Source: three-view drawing plus pictorial views. Frame: mm from the lowest corner of the part. A direction names the side the tool comes from. Give positions to 0.01 mm unless a question says otherwise; leave off trailing zeros. Loops run counter-clockwise (first coordinate to the right, second up) from the corner with the lowest first, then second, coordinate; pieces in that order, holes last. Notation, with made-up numbers: (22.5, -27) - (57.5, -27) arc R15 ccw to (57.5, -14) - close; hole circle Ø2 at (44.5, 10.25). An arc over 180 degrees is marked (long way). One line per item, written item: value.
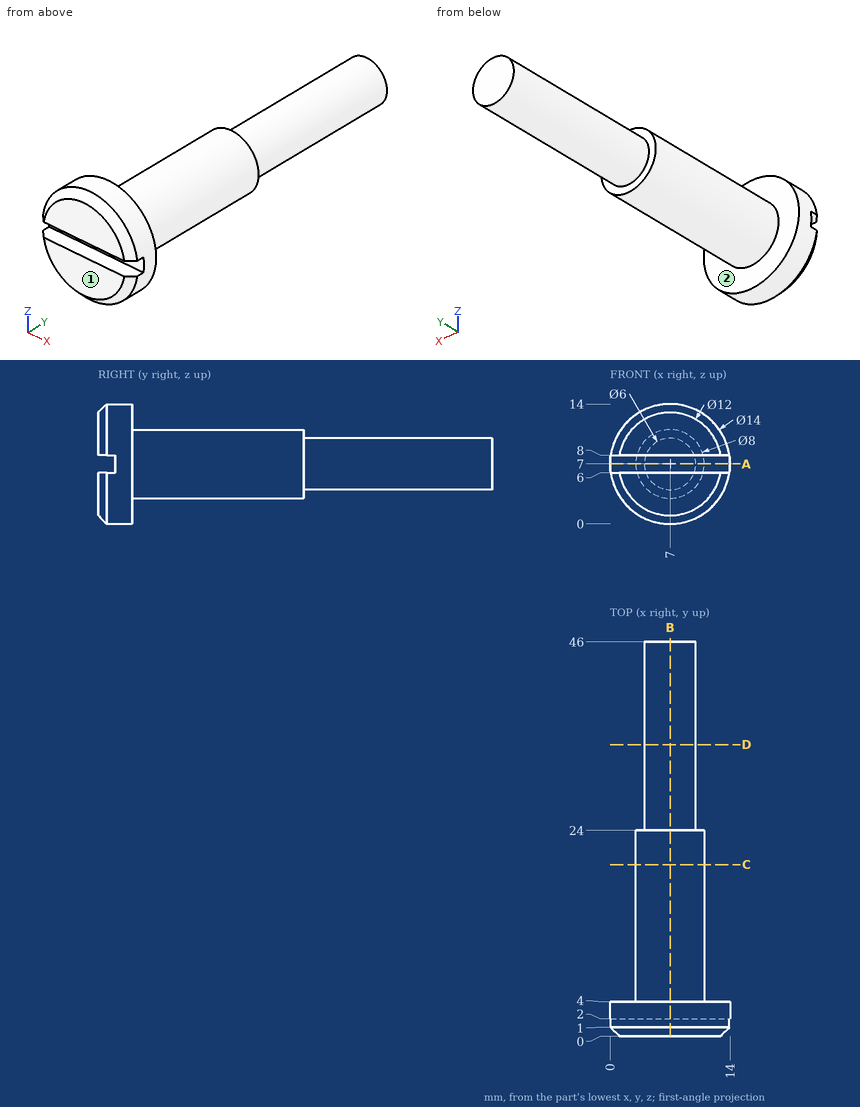
Item 1: Section C-C, the plane y = 20. Output: boundary loops of the cut face in (x, z).
Verdict:
outline: circle Ø8 at (7, 7)
Item 2: Section B-B, the plane x = 7. Output: boundary loops of the cut face in (y, z), and give its area (3 significant figures).
Verdict:
outline: (0, 1) - (1, 0) - (4, 0) - (4, 3) - (24, 3) - (24, 4) - (46, 4) - (46, 10) - (24, 10) - (24, 11) - (4, 11) - (4, 14) - (1, 14) - (0, 13) - (0, 8) - (2, 8) - (2, 6) - (0, 6) - close
area: 343 mm^2
Item 3: Section A-A, the plane z = 7. Output: boundary loops of the cut face in (x, y).
Verdict:
outline: (0, 2) - (14, 2) - (14, 4) - (11, 4) - (11, 24) - (10, 24) - (10, 46) - (4, 46) - (4, 24) - (3, 24) - (3, 4) - (0, 4) - close
Item 4: Material intervals for L1, parallel to Y at x = 3, z = 4.75; L2, parallel to Y at x = 6.75, z = 10.75; L3, parallel to X at y = 36.5, z = 6.75, sorted ascending.
Verdict:
L1: y = 0 to 4
L2: y = 0 to 24
L3: x = 4.01 to 9.99
Item 5: Pin query (flat end, axial travel): P1, Ø3, axis at x = 3.5, z = 3, coming from the -Y side; P2, Ø0.6, axis at x = 9, y = 1, coming from the +Z side; P3, Ø5, axis at x = 3.5, y = 13.5, coming from the -Z side; P4, Ø2, axis at x = 10.5, y = 1, coming from the -Z side. Return the tip coordinate at first contact, or that it passes through.
Verdict:
P1: stops at y = 0
P2: stops at z = 13.79
P3: stops at z = 3.13
P4: stops at z = 0.46
Item 6: Section D-D, the plane y = 34. Output: boundary loops of the cut face in (x, z).
Verdict:
outline: circle Ø6 at (7, 7)
Item 7: Access query for the marked faces 1 and 2. Directions: +Z, -Z, +X, -X, +Y, -Y. A direction counts if a zero-diameter tool reaches every point of the face in a straight line with its end or side. Return the directions, or none.
Verdict:
face 1: +Z, -Z, +X, -X, -Y
face 2: +Y
